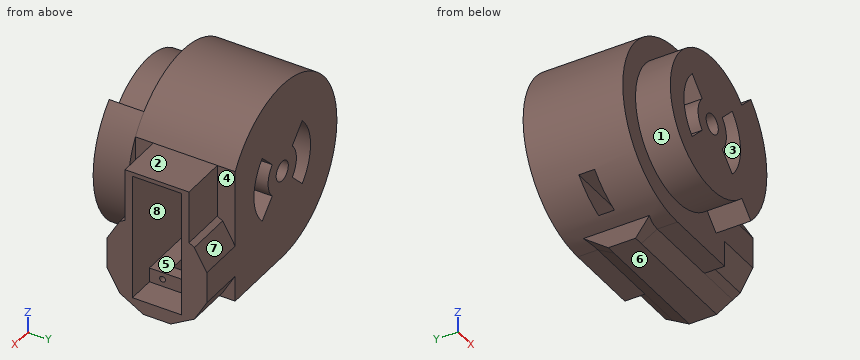
```python
from build123d import *

# Parameters (mm, degrees)
BOSS_EXTRUDE1_DEPTH     = 43
BOSS_EXTRUDE2_START     = 15
BOSS_EXTRUDE2_DEPTH     = 15
SKETCH5_W               = 42.2
SKETCH5_H               = 21.2
CUT_EXTRUDE1_DEPTH      = 41
SKETCH5_5_W             = 6.2
SKETCH5_5_H             = 21.2
SKETCH5_5_R             = 1.25
CUT_EXTRUDE2_DEPTH      = 12
SKETCH5_6_R             = 1.25
CUT_EXTRUDE3_DEPTH      = 35
CUT_EXTRUDE4_DEPTH      = 88.729655833
CUT_EXTRUDE4_DEPTH_BACK = 88.729655833
SKETCH6_R               = 4.3
CUT_EXTRUDE5_START      = -5
SKETCH7_W               = 10
SKETCH7_H               = 6.8
CUT_EXTRUDE5_DEPTH      = 94.632977309
CUT_EXTRUDE9_DEPTH      = 20
BOSS_EXTRUDE3_DEPTH     = 53.297297


with BuildPart() as part:
    # Sketch1 → Boss-Extrude1 (new body)
    with BuildSketch(Plane(origin=(0, 0, 0), x_dir=(1, 0, 0), z_dir=(0, 1, 0))):
        with BuildLine():
            Line((0, 38.625), (53.297297188, 38.625))
            Line((53.297297188, 38.625), (53.297297188, -19.575))
            Line((53.297297188, -19.575), (33.297297188, -19.575))
            ThreePointArc((33.297297188, -19.575), (-33.525922806, -19.180800948), (0, 38.625))
        make_face()
    extrude(amount=BOSS_EXTRUDE1_DEPTH)

    # Sketch4 → Boss-Extrude2 (add)
    with BuildSketch(Plane.XZ.offset(BOSS_EXTRUDE2_START)):
        with BuildLine():
            Line((20.948038393, 20.948038393), (27.311999423, 27.311999423))
            ThreePointArc((27.311999423, 27.311999423), (38.625, 0), (27.311999423, -27.311999423))
            Line((27.311999423, -27.311999423), (20.948038393, -20.948038393))
            ThreePointArc((20.948038393, -20.948038393), (-29.625, 0), (20.948038393, 20.948038393))
        make_face()
    extrude(amount=-BOSS_EXTRUDE2_DEPTH)

    # Sketch5 → Cut-Extrude1 (cut)
    with BuildSketch(Plane(origin=(53.297297188, 0, 0), x_dir=(0, 0, -1), z_dir=(1, 0, 0))):
        with Locations((9.525, 21.5)):
            Rectangle(SKETCH5_W, SKETCH5_H)
    extrude(amount=-CUT_EXTRUDE1_DEPTH, mode=Mode.SUBTRACT)

    # Sketch5<5> → Cut-Extrude2 (cut)
    # profile 1 of 2: a face of its own
    with BuildSketch(Plane(origin=(53.297297188, 0, 0), x_dir=(0, 0, -1), z_dir=(1, 0, 0))):
        with Locations((-14.675, 21.5)):
            Rectangle(SKETCH5_5_W, SKETCH5_5_H)
        with Locations((-14.575, 16.55)):
            Circle(SKETCH5_5_R, mode=Mode.SUBTRACT)
        with Locations((-14.575, 26.45)):
            Circle(SKETCH5_5_R, mode=Mode.SUBTRACT)
    # profile 2 of 2: a face of its own
    with BuildSketch(Plane(origin=(53.297297188, 0, 0), x_dir=(0, 0, -1), z_dir=(1, 0, 0))):
        with Locations((33.725, 21.5)):
            Rectangle(SKETCH5_5_W, SKETCH5_5_H)
        with Locations((33.625, 26.45)):
            Circle(SKETCH5_5_R, mode=Mode.SUBTRACT)
        with Locations((33.625, 16.55)):
            Circle(SKETCH5_5_R, mode=Mode.SUBTRACT)
    extrude(amount=-CUT_EXTRUDE2_DEPTH, mode=Mode.SUBTRACT)

    # Sketch5<6> → Cut-Extrude3 (cut)
    with BuildSketch(Plane(origin=(53.297297188, 0, 0), x_dir=(0, 0, -1), z_dir=(1, 0, 0))):
        with Locations((33.625, 26.45)):
            Circle(SKETCH5_6_R)
        with Locations((33.625, 16.55)):
            Circle(SKETCH5_6_R)
        with Locations((-14.575, 26.45)):
            Circle(SKETCH5_6_R)
        with Locations((-14.575, 16.55)):
            Circle(SKETCH5_6_R)
    extrude(amount=-CUT_EXTRUDE3_DEPTH, mode=Mode.SUBTRACT)

    # Sketch6 → Cut-Extrude4 (cut, two sides: drawn at the far end of the back side and taken through both)
    with BuildSketch(Plane.XZ.offset(15).offset(-CUT_EXTRUDE4_DEPTH_BACK)):
        with Locations(Location((0, 0, 0), (0, 0, 270))):
            Circle(SKETCH6_R)
        with BuildLine():
            Line((7.071067812, 7.071067812), (14.142135624, 14.142135624))
            ThreePointArc((14.142135624, 14.142135624), (20, 0), (14.142135624, -14.142135624))
            Line((14.142135624, -14.142135624), (7.071067812, -7.071067812))
            ThreePointArc((7.071067812, -7.071067812), (10, 0), (7.071067812, 7.071067812))
        make_face()
        with BuildLine():
            Line((-7.071067812, -7.071067812), (-14.142135624, -14.142135624))
            ThreePointArc((-14.142135624, -14.142135624), (-20, 0), (-14.142135624, 14.142135624))
            Line((-14.142135624, 14.142135624), (-7.071067812, 7.071067812))
            ThreePointArc((-7.071067812, 7.071067812), (-10, 0), (-7.071067812, -7.071067812))
        make_face()
    extrude(amount=CUT_EXTRUDE4_DEPTH + CUT_EXTRUDE4_DEPTH_BACK, mode=Mode.SUBTRACT)

    # Sketch7 → Cut-Extrude5 (cut, through all)
    with BuildSketch(Plane(origin=(41.297297188, 0, 0), x_dir=(0, 0, -1), z_dir=(1, 0, 0)).offset(CUT_EXTRUDE5_START)):
        with Locations((30.625, 21.5)):
            Rectangle(SKETCH7_W, SKETCH7_H)
    extrude(amount=-CUT_EXTRUDE5_DEPTH, mode=Mode.SUBTRACT)

    # Sketch9 → Cut-Extrude9 (cut)
    with BuildSketch(Plane(origin=(53.297297188, 0, 0), x_dir=(0, 0, -1), z_dir=(1, 0, 0))):
        Polygon((38.625, 43), (27.385907637, 43), (36.730117767, 37.605117767), (38.625, 34.323085464), align=None)
        Polygon((4.519882233, 37.605117767), (13.864092363, 43), (-19.575, 43), (-19.575, 35.3), (3.18902187, 35.3), align=None)
        Polygon((3.18902187, 7.7), (-19.575, 7.7), (-19.575, 0), (13.864092363, 0), (4.519882233, 5.394882233), align=None)
        Polygon((38.625, 0), (38.625, 8.676914536), (36.730117767, 5.394882233), (27.385907637, 0), align=None)
    extrude(amount=-CUT_EXTRUDE9_DEPTH, mode=Mode.SUBTRACT)

    # Sketch9<7> → Boss-Extrude3 (add)
    with BuildSketch(Plane(origin=(53.297297188, 0, 0), x_dir=(0, 0, -1), z_dir=(1, 0, 0))):
        Polygon((42.625, 27.394882233), (38.625, 34.323085464), (38.625, 8.676914536), (42.625, 15.605117767), align=None)
    extrude(amount=-BOSS_EXTRUDE3_DEPTH)

    # Chamfer1
    # the kernel refuses this chamfer: 10 mm, written as the material it adds along each edge
    with BuildSketch(Plane(origin=(1.88e-07, 57.509605692, -38.625), x_dir=(-0.9905263247652732, 0, 0.13732297676281435), z_dir=(0, -1, 0))) as chamfer1_piece_1_section:
        with BuildLine():
            Line((8.273915537, 0), (-1.522844477, 9.14873215))
            Line((-1.522844477, 9.14873215), (-1.720949742, 9.121267554))
            ThreePointArc((-1.720949742, 9.121267554), (-0.834678391, 4.564210108), (-0.198105265, -0.027464595))
            Line((-0.198105265, -0.027464595), (0.027464596, -0.198105265))
            ThreePointArc((0.027464596, -0.198105265), (4.132441209, 0.148053406), (8.26005162, -0.199518901))
            Line((8.26005162, -0.199518901), (8.273915537, 0))
        make_face()
    chamfer1_piece_1 = extrude(amount=72.019211383, mode=Mode.PRIVATE)
    chamfer1_piece_1 = split(chamfer1_piece_1, bisect_by=Plane(origin=(-3.347907706, 24.181861257, -44.480038526), z_dir=(0, -0.5000000000000007, 0.8660254037844383)), keep=Keep.TOP, mode=Mode.PRIVATE)
    chamfer1_piece_1 = split(chamfer1_piece_1, bisect_by=Plane(origin=(-3.347907706, 21.5, -42.625), z_dir=(0, 0, 1)), keep=Keep.TOP, mode=Mode.PRIVATE)
    chamfer1_piece_1 = split(chamfer1_piece_1, bisect_by=Plane(origin=(-3.347907706, 18.818138743, -44.480038526), z_dir=(0, 0.5000000000000001, 0.8660254037844386)), keep=Keep.TOP, mode=Mode.PRIVATE)
    add(chamfer1_piece_1)


solid = part.part
```
Verification items for the finished model (mm, model axes). Face numbers are marked on the shaded views. A direction names the side the tool comes from. Coordinates: 2 decimals unless noted, no trailing zeros. Loops run counter-clockwise (first coordinate to the right, second up) from the corner with the lowest first, then second, coordinate; pieces in that order, holes last. Notation, with made-up numbers: (1, 35) -> (48, 35) arc R21 ccw to (48, 51) -> close; hole circle Ø6 at (17, 25). An arc over 180 degrees is marked (long way). Put each result on its own line as item: value.
1. Section check A-A, the plane z = 0. Record the boundary of the cut face in (x, y) (3 decimals).
Result set:
outline: (-38.625, 0) -> (-29.625, 0) -> (-29.625, -15) -> (-20, -15) -> (-20, 43) -> (-38.625, 43) -> close; (-10, -15) -> (-4.3, -15) -> (-4.3, 43) -> (-10, 43) -> close; (4.3, -15) -> (10, -15) -> (10, 43) -> (4.3, 43) -> close; (20, -15) -> (38.625, -15) -> (38.625, 0) -> (33.297, 0) -> (33.297, 7.7) -> (53.297, 7.7) -> (53.297, 10.9) -> (20, 10.9) -> close; (20, 32.1) -> (53.297, 32.1) -> (53.297, 35.3) -> (33.297, 35.3) -> (33.297, 43) -> (20, 43) -> close
2. Gauge pin test, flat ends, axial feed: P1, Ø3, axis at x = 28.5, y = 16, coming from the +Z side; P2, Ø8, axis at x = 18.5, y = -6, coming from the -Z side; P3, Ø1.5, axis at y = 23.5, z = -10, coming from the +X side. Record the tip position at first contact, or that the pin passes through.
Result set:
P1: stops at z = 27.62
P2: stops at z = -25.83
P3: stops at x = 10.75
3. Thickness scan on line 1 (Z direction, x = 29, y = 26) (3 decimals); line 2 (X direction, y = 33, z = 14); line 3 (X direction, y = -11, z = 1). Record the ranges inside material, lowest first.
Result set:
line 1: z = -42.625 to -34.791, -32.459 to -30.625, 11.575 to 13.409, 15.741 to 25.513
line 2: x = -36 to -14.28, -14 to 14, 14.28 to 53.3
line 3: x = -29.61 to -19.97, -9.95 to -4.18, 4.18 to 9.95, 19.97 to 38.61
4. Section check B-B, the plane x = 44.5. Record the boundary of the cut face in (y, z) (3 decimals), then the cut area to 3 significant figures.
Result set:
outline: (0, -27.386) -> (5.395, -36.73) -> (15.605, -42.625) -> (27.395, -42.625) -> (37.605, -36.73) -> (43, -27.386) -> (43, -13.864) -> (37.605, -4.52) -> (35.3, -3.189) -> (35.3, 19.575) -> (7.7, 19.575) -> (7.7, -3.189) -> (5.395, -4.52) -> (0, -13.864) -> close; hole (10.9, -36.825) -> (32.1, -36.825) -> (32.1, 17.775) -> (10.9, 17.775) -> close
area: 924 mm^2
5. Section check C-C, the plane x = -22. Record the boundary of the cut face in (y, z) (3 decimals), then the cut area to 3 significant figures.
Result set:
outline: (-15, -19.84) -> (0, -19.84) -> (0, -31.747) -> (18.1, -31.747) -> (18.1, -25.625) -> (24.9, -25.625) -> (24.9, -31.747) -> (43, -31.747) -> (43, 31.747) -> (0, 31.747) -> (0, 19.84) -> (-15, 19.84) -> close
area: 3,280 mm^2
6. Tool access check on the marked faces 1, 2, 3 and 4. Record the directions out of +Z, -Z, +X, -X, +Y, -Y that give a thin tool (end or side, any length) a straight path to the whole face; none if there is none.
Result set:
face 1: -Y
face 2: +Z, +X, +Y, -Y
face 3: +Y, -Y
face 4: +Z, +X, +Y
7. Section check D-D, the plane z = -17. Record the boundary of the cut face in (x, y).
Result set:
outline: (-34.68, 0) -> (-24.26, 0) -> (-24.26, -15) -> (34.68, -15) -> (34.68, 0) -> (53.3, 0) -> (53.3, 10.9) -> (12.3, 10.9) -> (12.3, 32.1) -> (53.3, 32.1) -> (53.3, 43) -> (-34.68, 43) -> close
8. Mould release check, pull along Y, two halves, no side actions. Record for the marked faces 5, 6, 7 and 8: pulls with the +Y half, pulls with the -Y half, needs draft (parallel to the pull), parting line crosses it, or undercut.
Result set:
face 5: undercut
face 6: needs draft
face 7: pulls with the +Y half
face 8: undercut
